Read the model definition and answer for the solid it produces. Units are mm, in the model's axes. A direction names the side the tool comes from. Coordinates: 2 decimals unless noted, no trailing zeros. Order: outer loops, then holes, each group sorted by start corner. A loop starts at its lowest first (then second) coordinate and runs counter-clockwise, first axis right, second up. Notation, with made-up numbers: (10.5, -33.5) -> (33.5, -33.5) arc R7 cw to (33.5, -28.5) -> close; hole circle Ø7 at (79, 0.5). An arc over 180 degrees is marked (long way). Answer in a Markdown table with one row per item.
from build123d import *

# Parameters (mm, degrees)
F1_DEPTH = 25
F2_DEPTH = 51.4
F3_R     = 5
F4_DEPTH = 26
F5_DEPTH = 21
F6_R     = 5


with BuildPart() as f1:
    # F0 (on Top) → F1 (new body)
    with BuildSketch(Plane.XY):
        Polygon((-109.0911263708, -50.1850256925), (-69.0911263708, -90.1850256925), (90.9088736292, -90.1850256925), (90.9088736292, 79.8149743075), (90.9088736292, 82.8149743075), (50.9088736292, 122.8149743075), (-109.0911263708, 122.8149743075), align=None)
        with BuildLine():
            ThreePointArc((-55.0911263708, -39.4331600105), (-53.0729169233, -33.4089571938), (-47.8329224556, -29.8163749848))
            ThreePointArc((-47.8329224556, -29.8163749848), (1.5201909917, -0.7957829849), (30.5414983829, 48.5569097914))
            ThreePointArc((30.5414983829, 48.5569097914), (34.1340986973, 53.7968085215), (40.158243664, 55.8149743075))
            Line((40.158243664, 55.8149743075), (71.9088736292, 55.8149743075))
            ThreePointArc((71.9088736292, 55.8149743075), (78.979941441, 52.8860421194), (81.9088736292, 45.8149743075))
            Line((81.9088736292, 45.8149743075), (81.9088736292, -11.1850256925))
            ThreePointArc((81.9088736292, -11.1850256925), (78.979941441, -18.2560935043), (71.9088736292, -21.1850256925))
            Line((71.9088736292, -21.1850256925), (45.9088736292, -21.1850256925))
            ThreePointArc((45.9088736292, -21.1850256925), (28.9383108807, -28.214462944), (21.9088736292, -45.1850256925))
            Line((21.9088736292, -45.1850256925), (21.9088736292, -71.1850256925))
            ThreePointArc((21.9088736292, -71.1850256925), (18.979941441, -78.2560935043), (11.9088736292, -81.1850256925))
            Line((11.9088736292, -81.1850256925), (-45.0911263708, -81.1850256925))
            ThreePointArc((-45.0911263708, -81.1850256925), (-52.1621941827, -78.2560935043), (-55.0911263708, -71.1850256925))
            Line((-55.0911263708, -71.1850256925), (-55.0911263708, -39.4331600105))
        make_face(mode=Mode.SUBTRACT)
        with BuildLine():
            ThreePointArc((-25.2332619945, 93.9571099313), (3.3880299167, 93.6118592169), (2.3524786931, 65.0072235369))
            Line((2.3524786931, 65.0072235369), (-64.9455336496, -2.3237033734))
            ThreePointArc((-64.9455336496, -2.3237033734), (-93.2298044744, -2.3271608935), (-93.2332619945, 25.9571099313))
            Line((-93.2332619945, 25.9571099313), (-25.2332619945, 93.9571099313))
        make_face(mode=Mode.SUBTRACT)
        with BuildLine():
            ThreePointArc((30.5414983829, 48.5569097914), (1.5201909917, -0.7957829849), (-47.8329224556, -29.8163749848))
            ThreePointArc((-47.8329224556, -29.8163749848), (-53.0729169233, -33.4089571938), (-55.0911263708, -39.4331600105))
            Line((-55.0911263708, -39.4331600105), (-55.0911263708, -71.1850256925))
            ThreePointArc((-55.0911263708, -71.1850256925), (-52.1621941827, -78.2560935043), (-45.0911263708, -81.1850256925))
            Line((-45.0911263708, -81.1850256925), (11.9088736292, -81.1850256925))
            ThreePointArc((11.9088736292, -81.1850256925), (18.979941441, -78.2560935043), (21.9088736292, -71.1850256925))
            Line((21.9088736292, -71.1850256925), (21.9088736292, -45.1850256925))
            ThreePointArc((21.9088736292, -45.1850256925), (28.9383108807, -28.214462944), (45.9088736292, -21.1850256925))
            Line((45.9088736292, -21.1850256925), (71.9088736292, -21.1850256925))
            ThreePointArc((71.9088736292, -21.1850256925), (78.979941441, -18.2560935043), (81.9088736292, -11.1850256925))
            Line((81.9088736292, -11.1850256925), (81.9088736292, 45.8149743075))
            ThreePointArc((81.9088736292, 45.8149743075), (78.979941441, 52.8860421194), (71.9088736292, 55.8149743075))
            Line((71.9088736292, 55.8149743075), (40.158243664, 55.8149743075))
            ThreePointArc((40.158243664, 55.8149743075), (34.1340986973, 53.7968085215), (30.5414983829, 48.5569097914))
        make_face()
        with BuildLine():
            Line((-64.9455336496, -2.3237033734), (2.3524786931, 65.0072235369))
            ThreePointArc((2.3524786931, 65.0072235369), (3.3880299167, 93.6118592169), (-25.2332619945, 93.9571099313))
            Line((-25.2332619945, 93.9571099313), (-93.2332619945, 25.9571099313))
            ThreePointArc((-93.2332619945, 25.9571099313), (-93.2298044744, -2.3271608935), (-64.9455336496, -2.3237033734))
        make_face()
        with BuildLine():
            ThreePointArc((-72.020058559, 4.7439064957), (-86.1621941827, 4.7439064957), (-86.1621941827, 18.8860421194))
            Line((-86.1621941827, 18.8860421194), (-18.1621941827, 86.8860421194))
            ThreePointArc((-18.1621941827, 86.8860421194), (-4.020058559, 86.8860421194), (-4.020058559, 72.7439064957))
            Line((-4.020058559, 72.7439064957), (-72.020058559, 4.7439064957))
        make_face(mode=Mode.SUBTRACT)
        with BuildLine():
            Line((-18.1621941827, 86.8860421194), (-86.1621941827, 18.8860421194))
            ThreePointArc((-86.1621941827, 18.8860421194), (-86.1621941827, 4.7439064957), (-72.020058559, 4.7439064957))
            Line((-72.020058559, 4.7439064957), (-4.020058559, 72.7439064957))
            ThreePointArc((-4.020058559, 72.7439064957), (-4.020058559, 86.8860421194), (-18.1621941827, 86.8860421194))
        make_face()
    extrude(amount=F1_DEPTH)

    # F0 (on Top) → F2 (join)
    with BuildSketch(Plane.XY):
        with BuildLine():
            Line((-18.1621941827, 86.8860421194), (-86.1621941827, 18.8860421194))
            ThreePointArc((-86.1621941827, 18.8860421194), (-86.1621941827, 4.7439064957), (-72.020058559, 4.7439064957))
            Line((-72.020058559, 4.7439064957), (-4.020058559, 72.7439064957))
            ThreePointArc((-4.020058559, 72.7439064957), (-4.020058559, 86.8860421194), (-18.1621941827, 86.8860421194))
        make_face()
    extrude(amount=F2_DEPTH)

    # F3
    f3_edges = [f1.edges().sort_by_distance(p)[0] for p in [
        (-38.020059, 38.743906, 25),
    ]]
    fillet(f3_edges, radius=F3_R)

    # F0 (on Top) → F4 (join)
    with BuildSketch(Plane.XY):
        with BuildLine():
            ThreePointArc((30.5414983829, 48.5569097914), (1.5201909917, -0.7957829849), (-47.8329224556, -29.8163749848))
            ThreePointArc((-47.8329224556, -29.8163749848), (-53.0729169233, -33.4089571938), (-55.0911263708, -39.4331600105))
            Line((-55.0911263708, -39.4331600105), (-55.0911263708, -71.1850256925))
            ThreePointArc((-55.0911263708, -71.1850256925), (-52.1621941827, -78.2560935043), (-45.0911263708, -81.1850256925))
            Line((-45.0911263708, -81.1850256925), (11.9088736292, -81.1850256925))
            ThreePointArc((11.9088736292, -81.1850256925), (18.979941441, -78.2560935043), (21.9088736292, -71.1850256925))
            Line((21.9088736292, -71.1850256925), (21.9088736292, -45.1850256925))
            ThreePointArc((21.9088736292, -45.1850256925), (28.9383108807, -28.214462944), (45.9088736292, -21.1850256925))
            Line((45.9088736292, -21.1850256925), (71.9088736292, -21.1850256925))
            ThreePointArc((71.9088736292, -21.1850256925), (78.979941441, -18.2560935043), (81.9088736292, -11.1850256925))
            Line((81.9088736292, -11.1850256925), (81.9088736292, 45.8149743075))
            ThreePointArc((81.9088736292, 45.8149743075), (78.979941441, 52.8860421194), (71.9088736292, 55.8149743075))
            Line((71.9088736292, 55.8149743075), (40.158243664, 55.8149743075))
            ThreePointArc((40.158243664, 55.8149743075), (34.1340986973, 53.7968085215), (30.5414983829, 48.5569097914))
        make_face()
    extrude(amount=F4_DEPTH)

    # F5 (cut): a face of the model
    f5_faces = [f1.faces().sort_by_distance(p)[0] for p in [
        (17.7294443372, -17.0058627659, 26),
    ]]
    extrude(f5_faces, amount=-F5_DEPTH, mode=Mode.SUBTRACT)

    # F6
    f6_edges = [f1.edges().sort_by_distance(p)[0] for p in [
        (1.520191, -0.795783, 25),
        (1.520191, -0.795783, 5),
    ]]
    fillet(f6_edges, radius=F6_R)


solid = f1.part
Q1. The part is cut by section D-D (y = 103). Write down the section's boundary in (x, z).
Outcome:
| item | result |
|---|---|
| outline | (-109.09, 0) -> (70.72, 0) -> (70.72, 25) -> (-109.09, 25) -> close |
Q2. The part is cut by section A-A (z = 17.5). Write down the section's boundary in (x, y), then the cut area to 3 significant figures.
Outcome:
| item | result |
|---|---|
| outline | (-109.09, -50.19) -> (-69.09, -90.19) -> (90.91, -90.19) -> (90.91, 82.81) -> (50.91, 122.81) -> (-109.09, 122.81) -> close; hole (-55.09, -71.19) arc R10 ccw to (-45.09, -81.19) -> (11.91, -81.19) arc R10 ccw to (21.91, -71.19) -> (21.91, -45.19) arc R24 cw to (45.91, -21.19) -> (71.91, -21.19) arc R10 ccw to (81.91, -11.19) -> (81.91, 45.81) arc R10 ccw to (71.91, 55.81) -> (40.16, 55.81) arc R10 ccw to (30.54, 48.56) arc R114 cw to (-47.83, -29.82) arc R10 ccw to (-55.09, -39.43) -> close |
| area | 31,200 mm² |
Q3. For a pull along Y with two mould halves and no side action, classify faces 3 (the face through (-28, 122.815, 12)), 4 (the face through (-109.091, 38, 12)), 5 (the face through (-17, -81.185, 15)) as pulls with the +Y half, pulls with the -Y half, needs draft (parallel to the pull), parting line crosses it, or undercut.
Outcome:
| item | result |
|---|---|
| face 3 | pulls with the +Y half |
| face 4 | needs draft |
| face 5 | undercut |
Q4. The part is cut by section B-B (z = 43). Write down the section's boundary in (x, y), then the cut area to 3 significant figures.
Outcome:
| item | result |
|---|---|
| outline | (-86.16, 18.89) arc R10 ccw to (-72.02, 4.74) -> (-4.02, 72.74) arc R10 ccw to (-18.16, 86.89) -> close |
| area | 2,240 mm² |
Q5. For faces 1 (the face through (-52.749, 54.425, 26.426)), 2 (the face through (-56.59, -55.53, 23.57)), determine the directions among +Z, -Z, +X, -X, +Y, -Y from which every point of the face is accessible in a straight line to the end or side of a thin tool.
Outcome:
| item | result |
|---|---|
| face 1 | +Z, -X, +Y |
| face 2 | +Z |
Q6. Given pin 1 (10 mm diameter, centred on x = -20.5, y = 97, fed in from +Z); pin 2 (5 mm diameter, centred on y = -54, z = 17, fed in from -X); pin 3 (3 mm diameter, centred on x = 55, z = 12.5, fed in from +Y), each flat-ended and moving along its own axis, determine where each tip first touches the part or whether it passes through.
Outcome:
| item | result |
|---|---|
| pin 1 | z = 25.02 |
| pin 2 | x = -107.78 |
| pin 3 | y = 120.22 |
Q7. Consider line 1 (X direction, y = -40.5, z = 14.5); line 2 (Z direction, x = -93.5, y = 34.5); line 3 (X direction, y = -55.5, z = 7.5). Determine where each line is inside the solid, lowest interval first.
Outcome:
| item | result |
|---|---|
| line 1 | -109.09 to -55.09, 22.37 to 90.91 |
| line 2 | 0 to 25 |
| line 3 | -103.78 to -54.42, 21.24 to 90.91 |
Q8. The part is cut by section C-C (y = -64.5). Write down the section's boundary in (x, z), then the cut area to 3 significant figures.
Outcome:
| item | result |
|---|---|
| outline | (-94.78, 0) -> (90.91, 0) -> (90.91, 25) -> (26.91, 25) arc R5 ccw to (21.91, 20) -> (21.91, 10) arc R5 cw to (16.91, 5) -> (-50.09, 5) arc R5 cw to (-55.09, 10) -> (-55.09, 20) arc R5 ccw to (-60.09, 25) -> (-94.78, 25) -> close |
| area | 3,100 mm² |
